from build123d import *

# Parameters (mm, degrees)
F0_W     = 4
F0_H     = 2.5
F3_DEPTH = 2.5
F5_DEPTH = 2.5
F7_DEPTH = 2.5
F8_R     = 2
F9_R     = 2
F10_R    = 2
F11_R    = 2


with BuildPart() as f1:
    # F0 (on Front) → F1 (revolve)
    with BuildSketch(Plane.XZ):
        with Locations((29, 1.25)):
            Rectangle(F0_W, F0_H)
    revolve(axis=Axis((0, 0, 8.2326699048), (0, 0, 1)))



with BuildPart() as f3:
    # F2 (on Top) → F3 (new body, through all)
    with BuildSketch(Plane.XY):
        with BuildLine():
            Line((11.5, 16.2634559673), (-16.2634559673, 16.2634559673))
            Line((-16.2634559673, 16.2634559673), (-16.2634559673, 11.2634559673))
            Line((-16.2634559673, 11.2634559673), (-3, 11.2634559673))
            Line((-3, 11.2634559673), (-3, 2.5))
            Line((-3, 2.5), (-10, 2.5))
            Line((-10, 2.5), (-10, 5))
            Line((-10, 5), (-15, 5))
            Line((-15, 5), (-15, -5))
            Line((-15, -5), (-10, -5))
            Line((-10, -5), (-10, -2.5))
            Line((-10, -2.5), (-3, -2.5))
            Line((-3, -2.5), (-3, -11.2634559673))
            Line((-3, -11.2634559673), (-16.2634559673, -11.2634559673))
            Line((-16.2634559673, -11.2634559673), (-16.2634559673, -16.2634559673))
            Line((-16.2634559673, -16.2634559673), (11.5, -16.2634559673))
            ThreePointArc((11.5, -16.2634559673), (20.2343952269, -10.3062221039), (17.8764127782, 0))
            ThreePointArc((17.8764127782, 0), (20.2343952269, 10.3062221039), (11.5, 16.2634559673))
        make_face()
        with BuildLine():
            ThreePointArc((11.5, -2.5), (15.8817279836, -6.8817279836), (11.5, -11.2634559673))
            Line((11.5, -11.2634559673), (3, -11.2634559673))
            Line((3, -11.2634559673), (3, -2.5))
            Line((3, -2.5), (11.5, -2.5))
        make_face(mode=Mode.SUBTRACT)
        with BuildLine():
            Line((11.5, 2.5), (3, 2.5))
            Line((3, 2.5), (3, 11.2634559673))
            Line((3, 11.2634559673), (11.5, 11.2634559673))
            ThreePointArc((11.5, 11.2634559673), (15.8817279836, 6.8817279836), (11.5, 2.5))
        make_face(mode=Mode.SUBTRACT)
    extrude(amount=F3_DEPTH)

    # F4 (on face) → F5 (join, through all)
    with BuildSketch(Plane.XY.offset(2.5)):
        Polygon((-17.5, 9.5115462318), (-12.5, 9.5115462318), (-12.5, 11.2634559673), (-16.2634559673, 11.2634559673), (-16.2634559673, 16.2634559673), (-17.5, 16.2634559673), align=None)
        Polygon((-16.2634559673, -11.2634559673), (-12.5, -11.2634559673), (-12.5, -9.5115462318), (-17.5, -9.5115462318), (-17.5, -16.2634559673), (-16.2634559673, -16.2634559673), align=None)
    extrude(amount=-F5_DEPTH)


with BuildPart() as f1_1:
    add(f1.part)

    add(f3.part)  # F7 merges F3
    # F6 (on face) → F7 (join, through all)
    with BuildSketch(Plane.XY.offset(2.5)):
        with BuildLine():
            Line((-12.2809633628, 15.8164972687), (-17.2420989066, 20.7776328126))
            ThreePointArc((-17.2420989066, 20.7776328126), (-19.091883092, 19.091883092), (-20.7776328126, 17.2420989066))
            Line((-20.7776328126, 17.2420989066), (-15.8164972687, 12.2809633628))
            Line((-15.8164972687, 12.2809633628), (-12.2809633628, 15.8164972687))
        make_face()
        with BuildLine():
            ThreePointArc((20.7776328126, 17.2420989066), (19.091883092, 19.091883092), (17.2420989066, 20.7776328126))
            Line((17.2420989066, 20.7776328126), (11.4683862851, 15.0039201911))
            Line((11.4683862851, 15.0039201911), (15.0039201911, 11.4683862851))
            Line((15.0039201911, 11.4683862851), (20.7776328126, 17.2420989066))
        make_face()
        with BuildLine():
            ThreePointArc((17.2420989066, -20.7776328126), (19.091883092, -19.091883092), (20.7776328126, -17.2420989066))
            Line((20.7776328126, -17.2420989066), (15.277879572, -11.742345666))
            Line((15.277879572, -11.742345666), (11.742345666, -15.277879572))
            Line((11.742345666, -15.277879572), (17.2420989066, -20.7776328126))
        make_face()
        with BuildLine():
            Line((-15.6028734736, -12.0673543775), (-20.7776260963, -17.2421070001))
            ThreePointArc((-20.7776260963, -17.2421070001), (-19.091883092, -19.091883092), (-17.2421070001, -20.7776260963))
            Line((-17.2421070001, -20.7776260963), (-12.057121052, -15.5926401481))
            Line((-12.057121052, -15.5926401481), (-15.6028734736, -12.0673543775))
        make_face()
    extrude(amount=-F7_DEPTH)

    # F8
    f8_edges = [f1_1.edges().sort_by_distance(p)[0] for p in [
        (-17.242099, 20.777633, 1.25),
        (17.242099, 20.777633, 1.25),
    ]]
    fillet(f8_edges, radius=F8_R)

    # F9
    f9_edges = [f1_1.edges().sort_by_distance(p)[0] for p in [
        (-20.777633, 17.242099, 1.25),
        (-20.777626, -17.242107, 1.25),
    ]]
    fillet(f9_edges, radius=F9_R)

    # F10
    f10_edges = [f1_1.edges().sort_by_distance(p)[0] for p in [
        (-17.242107, -20.777626, 1.25),
        (17.242099, -20.777633, 1.25),
    ]]
    fillet(f10_edges, radius=F10_R)

    # F11
    f11_edges = [f1_1.edges().sort_by_distance(p)[0] for p in [
        (20.777633, 17.242099, 1.25),
        (20.777633, -17.242099, 1.25),
    ]]
    fillet(f11_edges, radius=F11_R)


solid = f1_1.part
Input: part model. Units: mm. Frame: model coordinates. Give positions to 0.01 mm unless a question says otherwise; leave off trailing zeros. Order: outer loops, then holes, each group sorted by start corner. A loop starts at its lowest first (then second) coordinate and runs counter-clockwise, first axis right, second up. Notation, with made-up numbers: (26, 69) - (42, 69) arc R11 cw to (42, 80) - close; hole circle Ø9 at (1, -34.75). An arc over 180 degrees is marked (long way). Answer as a JSON object with one key per item and string values. Group by question number.
Q1. Cut plane B-B, the plane x = 10. Output: boundary loops of the cut face in (y, z).
Q2. Line query: probe 1 along Y at (x, z) = (0.5, 1.95); probe 2 along X at (y, z) = (-10.5, 0.85); probe 3 along X at (y, z) = (-8.5, 0.6). Output: solid intervals per line, ascending.
Q3. Cut plane D-D, the plane z = 0.9. Count the separate pieces of the cut face and the enclosed holes in it, then the cut area to 3 significant figures.
Q4. Cut plane C-C, the plane y = -7.5. Output: boundary loops of the cut face in (x, z).
Q5. Cut plane A-A, the plane x = 0. Output: boundary loops of the cut face in (y, z).
Q6. Mould query, pull axis X, two halves, no side actions, for faces 1 (the face through (-4.036, 30.736, 1.268)), 2 (the face through (20.73, 16.2, 1.23)), 3 (the face through (0, 0, 0)), 4 (the face through (-15, 0, 1)). Classes: pulls with the +X half, pulls with the -X half, needs draft (parallel to the pull), parting line crosses it, or undercut.
Q7. First-contact query: pin 1 Ø0.8 at (y, z) = (-8.5, 1.5) entering from -X; pin 2 Ø1 at (y, z) = (-10, 1.5) entering from +X; pin 3 Ø0.9 at (y, z) = (10.5, 1) entering from +X; pin 4 Ø2 at (x, y) = (-24, 9) entering from +Z. Flat tips, straight axial feed; report the tip coordinate or a pass-through.
Results:
{
 "1": {"outline": "(-29.34, 0) - (-25.08, 0) - (-25.08, 2.5) - (-29.34, 2.5) - close; (-16.26, 0) - (-11.26, 0) - (-11.26, 2.5) - (-16.26, 2.5) - close; (-2.5, 0) - (2.5, 0) - (2.5, 2.5) - (-2.5, 2.5) - close; (11.26, 0) - (16.26, 0) - (16.26, 2.5) - (11.26, 2.5) - close; (25.08, 0) - (29.34, 0) - (29.34, 2.5) - (25.08, 2.5) - close"},
 "2": {"probe 1": "-31 to -27, -16.26 to 16.26, 27 to 31", "probe 2": "-29.17 to -24.87, -17.5 to -12.5, -3 to 3, 13.97 to 20.16, 24.87 to 29.17", "probe 3": "-29.81 to -25.63, -3 to 3, 15.57 to 20.74, 25.63 to 29.81"},
 "3": {"separate pieces": "1", "enclosed holes": "6", "area": "1,600 mm^2"},
 "4": {"outline": "(-30.08, 0) - (-25.94, 0) - (-25.94, 2.5) - (-30.08, 2.5) - close; (-3, 0) - (3, 0) - (3, 2.5) - (-3, 2.5) - close; (15.84, 0) - (20.86, 0) - (20.86, 2.5) - (15.84, 2.5) - close; (25.94, 0) - (30.08, 0) - (30.08, 2.5) - (25.94, 2.5) - close"},
 "5": {"outline": "(-31, 0) - (-27, 0) - (-27, 2.5) - (-31, 2.5) - close; (-16.26, 0) - (16.26, 0) - (16.26, 2.5) - (-16.26, 2.5) - close; (27, 0) - (31, 0) - (31, 2.5) - (27, 2.5) - close"},
 "6": {"face 1": "parting line crosses it", "face 2": "undercut", "face 3": "needs draft", "face 4": "undercut"},
 "7": {"pin 1": "x = -29.92", "pin 2": "x = 29.51", "pin 3": "x = 29.33", "pin 4": "through"}
}
